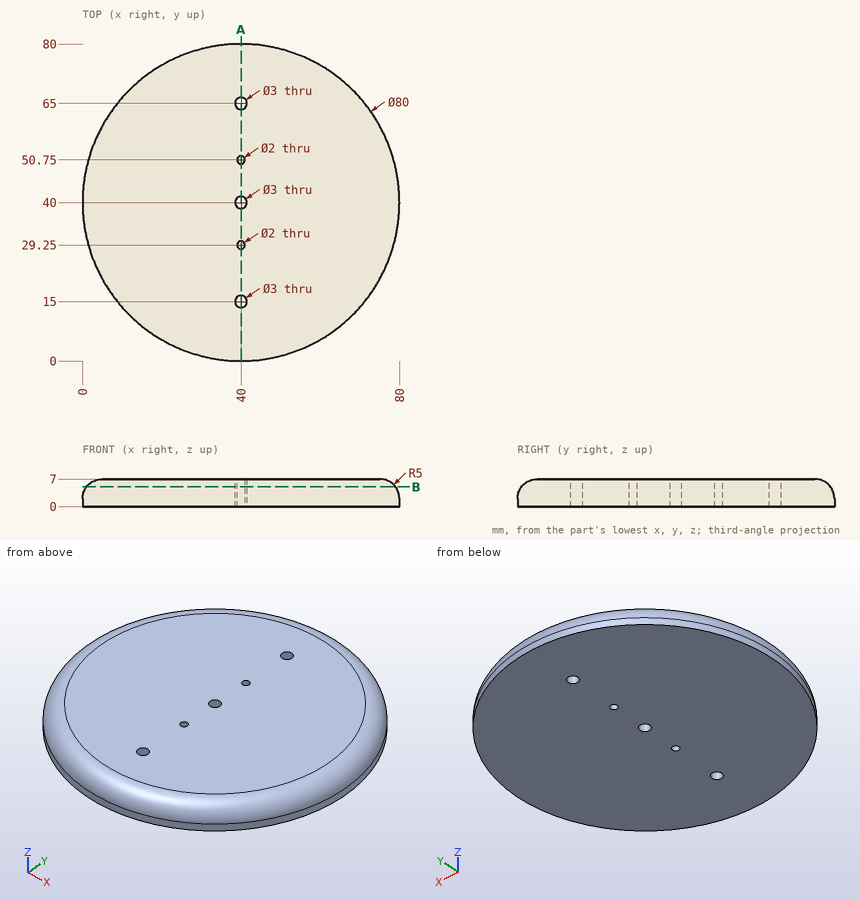
For this review, use the dimensioned drawing (mm, ordinates from the lowest corner) and the shaded views. Coordinates: 2 decimals unless noted, no trailing zeros. Write each loop counter-clockwise with the first axis right and the second up, starting at its lowest first coordinate (ties: lowest second). Pieces come first, ordered by that corner, then holes. Notation, with made-up numbers: (-35, 57) -> (-2, 57) arc R17 cw to (-2, 61) -> close; hole circle Ø6 at (38, 6.25). An arc over 180 degrees is marked (long way). Write each question's results on one line, items separated by ' | '. Start each with the question number.
(1) Take a section at B-B on z = 5. Write out the cut boundary in (x, y), and give its area (3 significant figures).
(2) Take a section at A-A on x = 40. Write out the cut boundary in (y, z), and give its area (3 significant figures).
(3) For line 1 along Y through (x, z) = (40, 2); line 2 along Y through (x, z) = (40, 6.5); line 3 along X through (y, z) = (65, 1.5), list the stretches that pass through material, from the lowest coordinate up. Write a range as from..to.
(4) Clearance check with flat-ended pins moving along their axes: P1, Ø1.8, axis at x = 40, y = 50.75, coming from the -Z side; P2, Ø1.5, axis at y = 47.5, z = 0.5, coming from the +X side; P3, Ø2, axis at x = 37.5, z = 3.5, coming from the -Y side. State where each tip first meets the part, or that it passes through.
Results found:
1) outline: circle Ø78 at (40, 40); hole circle Ø3 at (40, 15); hole circle Ø3 at (40, 40); hole circle Ø3 at (40, 65); hole circle Ø2 at (40, 29.25); hole circle Ø2 at (40, 50.75) | area: 4,750 mm2
2) outline: (0, 0) -> (13.5, 0) -> (13.5, 7) -> (5, 7) arc R5 ccw to (0, 2) -> close; (16.5, 0) -> (28.25, 0) -> (28.25, 7) -> (16.5, 7) -> close; (30.25, 0) -> (38.5, 0) -> (38.5, 7) -> (30.25, 7) -> close; (41.5, 0) -> (49.75, 0) -> (49.75, 7) -> (41.5, 7) -> close; (51.75, 0) -> (63.5, 0) -> (63.5, 7) -> (51.75, 7) -> close; (66.5, 0) -> (80, 0) -> (80, 2) arc R5 ccw to (75, 7) -> (66.5, 7) -> close | area: 458 mm2
3) line 1: y = 0..13.5, 16.5..28.25, 30.25..38.5, 41.5..49.75, 51.75..63.5, 66.5..80 | line 2: y = 2.82..13.5, 16.5..28.25, 30.25..38.5, 41.5..49.75, 51.75..63.5, 66.5..77.18 | line 3: x = 8.78..38.5, 41.5..71.22
4) P1: passes through | P2: stops at x = 79.43 | P3: stops at y = 0.09
